Answer from the drawing. Dimensions are ordinates in mm from the lowest x, y and z of the part. A direction names the side the tool comes from. Coordinates: 2 decimals unless noted, no trailing zeros. Write each loop counter-clockwise with the first axis right and the second up, starting at its lowest first coordinate (ties: lowest second). Pieces come first, ordered by that corner, then holes.
(1) Section D-D on z = 119.5 is taken. Write down the section's boundary in (x, y), then the cut area to 3 significant figures.
(2) Section B-B on y = 22 is taken. Write down the section's boundary in (x, z), then the cut area to 3 significant figures.
(3) Section C-C on x = 65 is taken. Write down the section's boundary in (y, z), then the cut area to 3 significant figures.
(4) Section A-A on y = 62 is taken. Write down the section's boundary in (x, z), then the cut area to 3 significant figures.
(5) Find the intervals of material crossed by probe 1 along Z at (x, y) = (80, 58); probe 2 along Y at (x, z) = (71, 185.5); probe 3 along Y at (x, z) = (15.5, 908), in increasing order.
(6) Given pin 1 (10.5 mm diameter, centred on x = 99.5, y = 41, fed in from +Z); pin 2 (1.5 mm diameter, centred on y = 76.5, z = 334.5, fed in from +X); pin 3 (8 mm diameter, centred on y = 75, z = 100, fed in from -X), each flat-ended and moving along its own axis, determine where each tip first touches the part or whether it passes through.
(7) Which of the six approach directions +Z, -Z, +X, -X, +Y, -Y give full straight-line access (tool end or side, diameter ignored) to the marked faces 1 and 2?
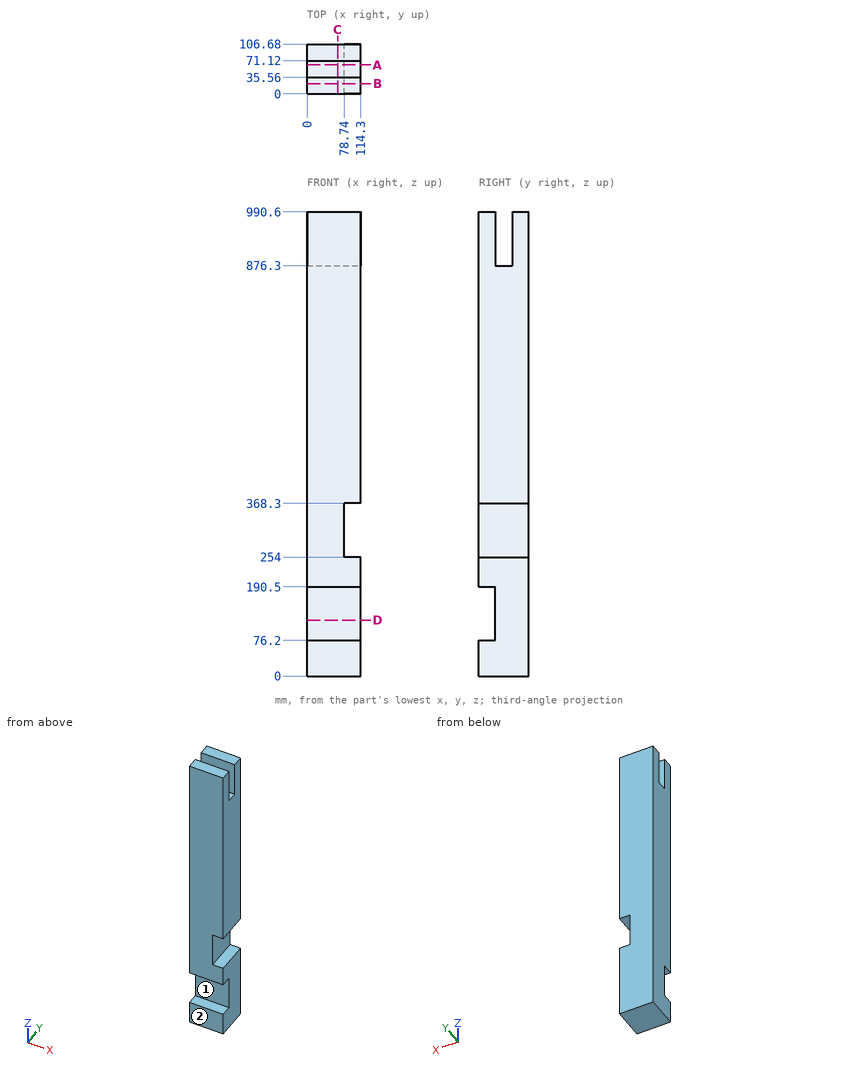
Response:
1. outline: (0, 35.56) - (114.3, 35.56) - (114.3, 106.68) - (0, 106.68) - close
1. area: 8,130 mm2
2. outline: (0, 0) - (114.3, 0) - (114.3, 76.2) - (0, 76.2) - close; (0, 190.5) - (114.3, 190.5) - (114.3, 254) - (78.74, 254) - (78.74, 368.3) - (114.3, 368.3) - (114.3, 990.6) - (0, 990.6) - close
2. area: 96,100 mm2
3. outline: (0, 0) - (106.68, 0) - (106.68, 990.6) - (71.12, 990.6) - (71.12, 876.3) - (35.56, 876.3) - (35.56, 990.6) - (0, 990.6) - (0, 190.5) - (35.56, 190.5) - (35.56, 76.2) - (0, 76.2) - close
3. area: 97,500 mm2
4. outline: (0, 0) - (114.3, 0) - (114.3, 254) - (78.74, 254) - (78.74, 368.3) - (114.3, 368.3) - (114.3, 876.3) - (0, 876.3) - close
4. area: 96,100 mm2
5. probe 1: z = 0 to 254, 368.3 to 876.3
5. probe 2: y = 35.56 to 106.68
5. probe 3: y = 0 to 35.56, 71.12 to 106.68
6. pin 1: stops at z = 876.3
6. pin 2: stops at x = 78.74
6. pin 3: stops at x = 0
7. face 1: +X, -X, -Y
7. face 2: +Z, -Z, +X, -X, -Y
